Geometry: final body of the model. Coordinates: model frame, mm. Face numbers are marked on the shaded views. Give positions to 0.01 mm unless a question says otherwise; leave off trailing zeros. Order: outer loops, then holes, each group sorted by start corner. A loop starts at its lowest first (then second) coordinate and runs counter-clockwise, first axis right, second up. Notation, with made-up numbers: (27, 64) - (73, 64) arc R32 ccw to (73, 103) - close; hole circle Ø2 at (25.25, 41.5). An arc over 180 degrees is marked (long way). Put each result on its own line as item: value. Start each with the question number.
1. Section C-C on y = -2.5. Return the cut outline in (x, z), plus the area to 3 significant figures.
2. Section D-D on z = -15. Return the cut outline in (x, y), plus the area to 3 significant figures.
3. Mould query, pull axis Z, two halves, no side actions, for the marked faces 1 and 2. Classes: pulls with the +Z half, pulls with the -Z half, needs draft (parallel to the pull), parting line crosses it, or undercut.
4. First-contact query: P1, Ø0.6, axis at y = 0, z = 0, coming from the +X side; P2, Ø2, axis at x = 4.5, y = 3, coming from the +Z side; P3, Ø1.9, axis at y = -2, z = -41, coming from the -X side. Flat tips, straight axial feed; report the tip coordinate or a pass-through.
5. Ray query, line 1 along Y through (x, z) = (2.75, -40); line 2 along Z through (x, y) = (2.25, 0.25); line 3 along Y through (x, z) = (3.3, 0). Return the intervals inside material, ascending. Write a range as from..to.
6. Section B-B on y = 1.25. Return the cut outline in (x, z), plus the area to 3 significant figures.
7. Section A-A on x = 2. Return the cut outline in (y, z), plus the area to 3 significant figures.
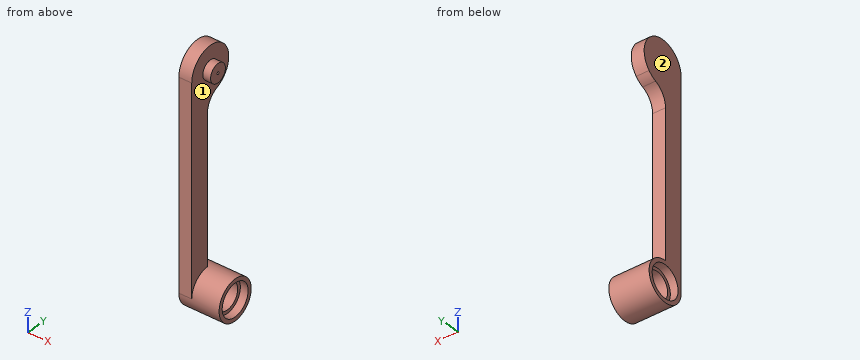
from build123d import *

# Parameters (mm, degrees)
SKETCH_1_R               = 4.5
SKETCH_1_W               = 43.9
SKETCH_1_H               = 7.8
EXTRUDE_1_DEPTH          = 2.5
EXTRUDE_START            = 2.5
SKETCH_1_6_R             = 1.8
SKETCH_1_6_R_2           = 0.25
EXTRUDE_3_DEPTH          = 1.5
SKETCH_1_5_W             = 7.8
SKETCH_1_5_H             = 7.8
EXTRUDE_2_DEPTH          = 7.8
SKETCH_1_7_R             = 2.5
CUT_EXTRUDE_1_DEPTH      = 45.814060294
SKETCH_1_8_R             = 3.15
SKETCH_1_8_R_2           = 2.5
CUT_EXTRUDE_2_DEPTH      = 1.5
CUT_EXTRUDE_START        = 6.3
SKETCH_1_9_R             = 3.15
SKETCH_1_9_R_2           = 2.5
CUT_EXTRUDE_3_DEPTH      = 1.5
CUT_EXTRUDE_4_DEPTH      = 45.814060294
FILLET_1_R               = 3.9
CUT_EXTRUDE_5_DEPTH      = 51.552448012
CUT_EXTRUDE_5_DEPTH_BACK = 51.552448012
SKETCH_3_W               = 64.704037325
SKETCH_3_H               = 20.946447886


with BuildPart() as part:
    # 草图1 → 凸台-拉伸1 (new body)
    with BuildSketch(Plane(origin=(0, 0, 0), x_dir=(0, 0, -1), z_dir=(1, 0, 0))):
        Circle(SKETCH_1_R)
        with Locations((21.95, -0.6)):
            Rectangle(SKETCH_1_W, SKETCH_1_H)
    extrude(amount=EXTRUDE_1_DEPTH)

    # 草图1<6> → 凸台-拉伸3 (add)
    with BuildSketch(Plane(origin=(0, 0, 0), x_dir=(0, 0, -1), z_dir=(1, 0, 0)).offset(EXTRUDE_START)):
        Circle(SKETCH_1_6_R)
        Circle(SKETCH_1_6_R_2, mode=Mode.SUBTRACT)
    extrude(amount=EXTRUDE_3_DEPTH)

    # 草图1<5> → 凸台-拉伸2 (add)
    with BuildSketch(Plane(origin=(0, 0, 0), x_dir=(0, 0, -1), z_dir=(1, 0, 0))):
        with Locations((40, -0.6)):
            Rectangle(SKETCH_1_5_W, SKETCH_1_5_H)
    extrude(amount=EXTRUDE_2_DEPTH)

    # 草图1<7> → 切除-拉伸1 (cut, through all)
    with BuildSketch(Plane(origin=(0, 0, 0), x_dir=(0, 0, -1), z_dir=(1, 0, 0))):
        with Locations((40, -0.6)):
            Circle(SKETCH_1_7_R)
    extrude(amount=CUT_EXTRUDE_1_DEPTH, mode=Mode.SUBTRACT)

    # 草图1<8> → 切除-拉伸2 (cut)
    with BuildSketch(Plane(origin=(0, 0, 0), x_dir=(0, 0, -1), z_dir=(1, 0, 0))):
        with Locations((40, -0.6)):
            Circle(SKETCH_1_8_R)
        with Locations((40, -0.6)):
            Circle(SKETCH_1_8_R_2, mode=Mode.SUBTRACT)
    extrude(amount=CUT_EXTRUDE_2_DEPTH, mode=Mode.SUBTRACT)

    # 草图1<9> → 切除-拉伸3 (cut)
    with BuildSketch(Plane(origin=(0, 0, 0), x_dir=(0, 0, -1), z_dir=(1, 0, 0)).offset(CUT_EXTRUDE_START)):
        with Locations((40, -0.6)):
            Circle(SKETCH_1_9_R)
        with Locations((40, -0.6)):
            Circle(SKETCH_1_9_R_2, mode=Mode.SUBTRACT)
    extrude(amount=CUT_EXTRUDE_3_DEPTH, mode=Mode.SUBTRACT)

    # 草图2 → 切除-拉伸4 (cut, through all)
    with BuildSketch(Plane.ZY):
        Polygon((-4.5, 3.3), (-36.1, 3.3), (-36.1, -0.7), (-4.5, -0.7), (-4.5, 0), align=None)
        with BuildLine():
            Line((-3.059411708, 3.3), (-4.5, 3.3))
            Line((-4.5, 3.3), (-4.5, 0))
            ThreePointArc((-4.5, 0), (-4.124157653, 1.800367645), (-3.059411708, 3.3))
        make_face()
    extrude(amount=-CUT_EXTRUDE_4_DEPTH, mode=Mode.SUBTRACT)

    # 圆角1
    # the kernel refuses this fillet: 3.9 mm, written as the material it adds along each edge
    with BuildSketch(Plane(origin=(0, -0.7, -4.5), x_dir=(0, 0, -1), z_dir=(1, 0, 0))) as fillet_1_piece_1:
        with BuildLine():
            CenterArc((3.266595136, 3.9), FILLET_1_R, 202.392687805, 67.607312195)
            Line((-0.339324035, 2.414285714), (-0.699915952, 2.265714286))
            ThreePointArc((-0.699915952, 2.265714286), (-0.39, 0.7), (-0.39, 0))
            Line((-0.39, 0), (0, -0.39))
            Line((0, -0.39), (3.266595136, -0.39))
            Line((3.266595136, -0.39), (3.266595136, 0))
        make_face()
    extrude(amount=2.5)
    # the kernel refuses this fillet: 3.9 mm, written as the material it takes off along each edge
    with BuildSketch(Plane(origin=(-9.75, -4.5, -43.9), x_dir=(0, 1, 0), z_dir=(1, 0, 0))) as fillet_1_2_piece_1:
        with BuildLine():
            CenterArc((FILLET_1_R, FILLET_1_R), FILLET_1_R, 180, 90)
            Line((0, FILLET_1_R), (0, 0))
            Line((0, 0), (FILLET_1_R, 0))
        make_face()
    extrude(amount=27.3, mode=Mode.SUBTRACT)
    with BuildSketch(Plane(origin=(17.55, 3.3, -43.9), x_dir=(0, 0, 1), z_dir=(-1, 0, 0)), Plane(origin=(17.55, 3.3, -36.1), x_dir=(0, -1, 0), z_dir=(-1, 0, 0))) as fillet_1_2_piece_2:
        with BuildLine():
            CenterArc((FILLET_1_R, -FILLET_1_R), FILLET_1_R, 90, 90)
            Line((0, -FILLET_1_R), (0, 0))
            Line((0, 0), (FILLET_1_R, 0))
        make_face()
    extrude(amount=27.3, mode=Mode.SUBTRACT)
    with BuildSketch(Plane(origin=(-7.25, -4.5, -36.1), x_dir=(0, 1, 0), z_dir=(1, 0, 0))) as fillet_1_2_piece_3_section:
        with BuildLine():
            CenterArc((FILLET_1_R, -FILLET_1_R), FILLET_1_R, 90, 90)
            Line((0, -FILLET_1_R), (0, 0))
            Line((0, 0), (FILLET_1_R, 0))
        make_face()
    fillet_1_2_piece_3 = extrude(amount=24.8, mode=Mode.PRIVATE)
    fillet_1_2_piece_3 = split(fillet_1_2_piece_3, bisect_by=Plane(origin=(1.25, -0.7, -36.100384668), z_dir=(0, 1, 0)), keep=Keep.TOP, mode=Mode.PRIVATE)
    add(fillet_1_2_piece_3, mode=Mode.SUBTRACT)
    with BuildSketch(Plane(origin=(2.5, -4.5, -36.1), x_dir=(0, 1, 0), z_dir=(1, 0, 0))) as fillet_1_2_piece_4:
        with BuildLine():
            CenterArc((FILLET_1_R, -FILLET_1_R), FILLET_1_R, 90, 90)
            Line((0, -FILLET_1_R), (0, 0))
            Line((0, 0), (FILLET_1_R, 0))
        make_face()
    extrude(amount=15.05, mode=Mode.SUBTRACT)


with BuildPart() as body_2:
    # 镜向2: mirrored copy
    add(part.part.mirror(Plane.ZX.offset(-10)))

    # 草图3 → 切除-拉伸5 (cut, two sides: drawn at the far end of the back side and taken through both)
    with BuildSketch(Plane(origin=(2.5, 0, 0), x_dir=(0, 0, -1), z_dir=(1, 0, 0)).offset(-CUT_EXTRUDE_5_DEPTH_BACK)):
        with Locations((21.266459283, -20.282495136)):
            Rectangle(SKETCH_3_W, SKETCH_3_H)
    extrude(amount=CUT_EXTRUDE_5_DEPTH + CUT_EXTRUDE_5_DEPTH_BACK, mode=Mode.SUBTRACT)


solid = part.part
Resolved:
1. outline: (0, -43.41) - (7.8, -43.41) - (7.8, -42.51) - (6.3, -42.51) - (6.3, -41.62) - (1.5, -41.62) - (1.5, -42.51) - (0, -42.51) - close; (0, -37.49) - (1.5, -37.49) - (1.5, -38.38) - (6.3, -38.38) - (6.3, -37.49) - (7.8, -37.49) - (7.8, -36.59) - (2.5, -36.59) - (2.5, 3.74) - (0, 3.74) - close
1. area: 123 mm^2
2. outline: (0, -4.5) - (2.5, -4.5) - (2.5, -0.7) - (0, -0.7) - close
2. area: 9.50 mm^2
3. face 1: undercut
3. face 2: needs draft
4. P1: x = 4
4. P2: z = -37.09
4. P3: x = 1.5
5. line 1: -4.5..-3.1, 1.9..3.3
5. line 2: -43.81..-42.35, -37.65..-36.19, -5.22..4.49
5. line 3: -1.8..-0.25, 0.25..1.8
6. outline: (0, -43.43) - (7.8, -43.43) - (7.8, -42.55) - (6.3, -42.55) - (6.3, -41.68) - (1.5, -41.68) - (1.5, -42.55) - (0, -42.55) - close; (0, -37.45) - (1.5, -37.45) - (1.5, -38.32) - (6.3, -38.32) - (6.3, -37.45) - (7.8, -37.45) - (7.8, -36.57) - (0, -36.57) - close; (0, -4.39) - (2.5, -4.39) - (2.5, -1.3) - (4, -1.3) - (4, 1.3) - (2.5, 1.3) - (2.5, 4.32) - (0, 4.32) - close
6. area: 47.8 mm^2
7. outline: (-4.5, -40) arc R3.9 ccw (long way) to (-0.7, -36.1) - (-0.7, -7.77) arc R3.9 cw to (1.71, -4.16) arc R4.5 ccw (long way) to (-4.5, 0) - close; hole circle Ø5 at (-0.6, -40)
7. area: 221 mm^2
